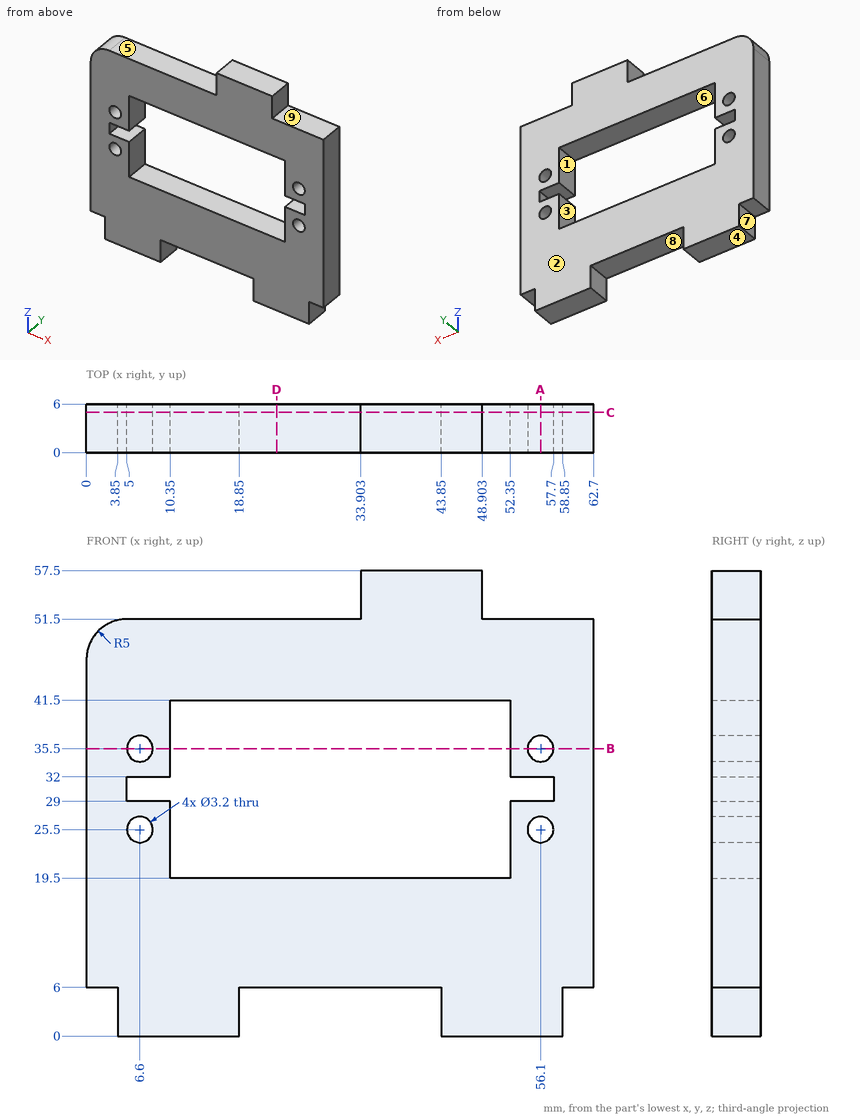
Design review of the part shown in the three views and the two pictorial views. Dimensions are in mm from the part's minimum x, y and z. A direction names the side the tool comes from. Give positions to 0.01 mm unless a question says otherwise; leave off trailing zeros. Loops run counter-clockwise (first coordinate to the right, second up) from the corner with the lowest first, then second, coordinate; pieces in that order, holes last. Notation, with made-up numbers: (82.25, 4) -> (126.25, 4) arc R19 cw to (126.25, 16) -> close; hole circle Ø5 at (23.5, 19). An arc over 180 degrees is marked (long way). One line per question, with ' | ' between items.
1) For the marked faces 5, 6, 7, 8 and 9, list the 3-axis set-ups (+Z, -Z, +X, -X, +Y, -Y) from which the entire face can be reached by the end or side of a thin tool; tool diameter is ignored.
Resolved:
face 5: +Z, -X, +Y, -Y | face 6: +Y, -Y | face 7: -Z, -X, +Y, -Y | face 8: -Z, +Y, -Y | face 9: +Z, +X, +Y, -Y
2) We need section D-D (x = 23.5). Write out the cut boundary in (y, z), plus the area to 3 significant figures.
Resolved:
outline: (0, 6) -> (6, 6) -> (6, 19.5) -> (0, 19.5) -> close; (0, 41.5) -> (6, 41.5) -> (6, 51.5) -> (0, 51.5) -> close | area: 141 mm2
3) The part is to be moulded in two halves that separate along Z. For the marked faces 1, 2, 3 and 4, say which applies: +Z half, -Z half, draft (parallel to the pull), parting line (faces both ways), or undercut.
Resolved:
face 1: undercut | face 2: draft | face 3: undercut | face 4: -Z half
4) We need section B-B (z = 35.5). Write out the cut boundary in (x, y).
Resolved:
outline: (0, 0) -> (5, 0) -> (5, 6) -> (0, 6) -> close; (8.2, 0) -> (10.35, 0) -> (10.35, 6) -> (8.2, 6) -> close; (52.35, 0) -> (54.5, 0) -> (54.5, 6) -> (52.35, 6) -> close; (57.7, 0) -> (62.7, 0) -> (62.7, 6) -> (57.7, 6) -> close
5) We need section A-A (x = 56.1). Write out the cut boundary in (y, z).
Resolved:
outline: (0, 0) -> (6, 0) -> (6, 23.9) -> (0, 23.9) -> close; (0, 27.1) -> (6, 27.1) -> (6, 29) -> (0, 29) -> close; (0, 32) -> (6, 32) -> (6, 33.9) -> (0, 33.9) -> close; (0, 37.1) -> (6, 37.1) -> (6, 51.5) -> (0, 51.5) -> close
6) Insertion check: pin 1 Ø3 at (x, y) = (1.5, 4) entering from -Z; pin 2 Ø1.8 at (y, z) = (3.5, 3.5) entering from -X. Each pin has a flat end and moves straight along its axis. Give the tip position at first contact, or say it passes through.
Resolved:
pin 1: stops at z = 6 | pin 2: stops at x = 3.85
7) To check wall thickness, follow probe 1 along Z at (x, y) = (56.1, 3.65); probe 2 along Z at (x, y) = (52, 5.4); probe 3 along X at (y, z) = (2.35, 28). State the ranges of each line that lie inside material, in increasing order.
Resolved:
probe 1: z = 0 to 23.9, 27.1 to 29, 32 to 33.9, 37.1 to 51.5 | probe 2: z = 0 to 19.5, 41.5 to 51.5 | probe 3: x = 0 to 10.35, 52.35 to 62.7
8) We need section C-C (y = 4.95). Give the number of separate pieces and of enclosed holes in the cut face, plus the area to 3 significant figures.
Resolved:
separate pieces: 1 | enclosed holes: 5 | area: 2,130 mm2
